Design review of the part built by this model. Coordinates are the model's own, in mm. A direction names the side the tool comes from. Give positions to 0.01 mm unless a question says otherwise; leave off trailing zeros. Write each loop counter-clockwise with the first axis right and the second up, starting at its lowest first coordinate (ties: lowest second). Pieces come first, ordered by that corner, then holes. Notation, with made-up numbers: M -16,19 L -11,19 A18 ccw -11,25 Z; hole C -31.5,32.25 d11. An arc over 180 degrees is marked long. Answer in a Markdown table with one row per item.
```python
from build123d import *

# Parameters (mm, degrees)
SKETCH1_W           = 15
SKETCH1_H           = 85
SKETCH1_R           = 1.5
BOSS_EXTRUDE1_DEPTH = 2
SKETCH2_R           = 5
CUT_EXTRUDE1_DEPTH  = 0.5
FILLET1_R           = 1


with BuildPart() as part:
    # Sketch1 → Boss-Extrude1 (new body)
    with BuildSketch(Plane(origin=(0, 0, 0), x_dir=(1, 0, 0), z_dir=(0, 1, 0))):
        with Locations((7.5, 42.5)):
            Rectangle(SKETCH1_W, SKETCH1_H)
        with Locations(Location((7.5, 70.5, 0), (0, 0, 270))):
            Circle(SKETCH1_R, mode=Mode.SUBTRACT)
        with Locations(Location((7.5, 5.5, 0), (0, 0, 270))):
            Circle(SKETCH1_R, mode=Mode.SUBTRACT)
    extrude(amount=BOSS_EXTRUDE1_DEPTH)

    # Sketch2 → Cut-Extrude1 (cut)
    with BuildSketch(Plane(origin=(0, 2, 0), x_dir=(1, 0, 0), z_dir=(0, 1, 0))):
        with Locations(Location((7.5, 70.5, 0), (0, 0, 270))):
            Circle(SKETCH2_R)
    extrude(amount=-CUT_EXTRUDE1_DEPTH, mode=Mode.SUBTRACT)

    # Fillet1
    fillet1_edges = [part.edges().sort_by_distance(p)[0] for p in [
        (0, 1, -85),
        (15, 1, -85),
        (15, 1, 0),
        (0, 1, 0),
    ]]
    fillet(fillet1_edges, radius=FILLET1_R)


solid = part.part
```
1) For faces 4 (the face through (6, 1.5, -72)), 5 (the face through (7, 2, -43)), list the 3-axis set-ups (+Z, -Z, +X, -X, +Y, -Y) from which the entire face can be reached by the end or side of a thin tool; tool diameter is ignored.
Geometry says:
| item | result |
|---|---|
| face 4 | +Y |
| face 5 | +Z, -Z, +X, -X, +Y |
2) Add section A-A (z = -70.5). Write out the cut boundary in (x, y), and give its area (3 significant figures).
Geometry says:
| item | result |
|---|---|
| outline | M 0,0 L 6,0 L 6,1.5 L 2.5,1.5 L 2.5,2 L 0,2 Z; M 9,0 L 15,0 L 15,2 L 12.5,2 L 12.5,1.5 L 9,1.5 Z |
| area | 20.5 mm^2 |
3) The part is to be moulded in two halves that separate along X. For faces 1 (the face through (0, 1, -42)), 2 (the face through (7, 1, -85)), 3 (the face through (6.925, 0.74, -69.114)), say which applies: released by +X, released by -X, zero draft, split by the parting line, or undercut.
Geometry says:
| item | result |
|---|---|
| face 1 | released by -X |
| face 2 | zero draft |
| face 3 | undercut |
4) Insertion check: P1, Ø2.5, axis at x = 7.5, z = -5.5, coming from the -Y side (1 decimal); P2, Ø5, axis at x = 8.5, z = -70.5, coming from the +Y side. Each pin has a flat end and moves straight along its axis. Give the tip position at first contact, or say it passes through.
Geometry says:
| item | result |
|---|---|
| P1 | through |
| P2 | y = 1.5 |
5) Add section C-C (x = 11.5). Write out the cut boundary in (y, z), and give its area (3 significant figures).
Geometry says:
| item | result |
|---|---|
| outline | M 0,-85 L 2,-85 L 2,-73.5 L 1.5,-73.5 L 1.5,-67.5 L 2,-67.5 L 2,0 L 0,0 Z |
| area | 167 mm^2 |
6) Add section B-B (x = 7.5). Write out the cut boundary in (y, z), and give its area (4 significant figures).
Geometry says:
| item | result |
|---|---|
| outline | M 0,-85 L 2,-85 L 2,-75.5 L 1.5,-75.5 L 1.5,-72 L 0,-72 Z; M 0,-69 L 1.5,-69 L 1.5,-65.5 L 2,-65.5 L 2,-7 L 0,-7 Z; M 0,-4 L 2,-4 L 2,0 L 0,0 Z |
| area | 154.5 mm^2 |
7) To check wall thickness, follow probe 1 along X at (y, z) = (1.85, -70.5); probe 2 along Z at (x, y) = (8.75, 0.95); probe 3 along X at (y, z) = (1.45, -5.5). State the ranges of each line that lie inside material, in increasing order. Write a range as [from, to].
Geometry says:
| item | result |
|---|---|
| probe 1 | [0, 2.5], [12.5, 15] |
| probe 2 | [-85, -71.33], [-69.67, -6.33], [-4.67, 0] |
| probe 3 | [0, 6], [9, 15] |
8) Add section D-D (z = -5.5). Write out the cut boundary in (x, y), and give its area (3 significant figures).
Geometry says:
| item | result |
|---|---|
| outline | M 0,0 L 6,0 L 6,2 L 0,2 Z; M 9,0 L 15,0 L 15,2 L 9,2 Z |
| area | 24.0 mm^2 |
